Could you check a few things on this drawing? It's one solid part, dimensions in mm from its lowest x, y, z. Coordinates: 2 decimals unless noted, no trailing zeros. Loops run counter-clockwise (first coordinate to the right, second up) from the corner with the lowest first, then second, coordinate; pieces in that order, holes last. Notation, with made-up numbers: M 68,4.5 L 101,4.5 A32 ccw 101,33.5 Z; hole C 60,31 d11. An arc over 180 degrees is marked long. Answer as a JSON object with one key per item and string values. Group by question number.
Item 1: If I drill on line 1 (X direction, y = 26.5, z = 8.5); line 2 (Y direction, x = 201.5, z = 6); line 3 (Z direction, x = 217.5, y = 18.5), over which ranges is the centre line in solid material (lowest first)?
Item 2: Suppose I cut it at A-A (y = 29). Write out the boundary of the cut face in (x, z), then the cut area to 3 significant figures.
Item 3: Suppose I cut it at C-C (x = 96.5). Write out the boundary of the cut face in (y, z), then the cut area to 3 significant figures.
Item 4: Suppose I cut it at B-B (y = 6). Write out the boundary of the cut face in (x, z).
Item 5: Suppose I cut it at D-D (z = 38). Write out the boundary of the cut face in (x, y), then the cut area to 3 significant figures.
Item 6: I'm going to push flat-ended pins straight in: pin 1 Ø3 at (x, y) = (274.5, 12) entering from -Z; pin 2 Ø6 at (x, z) = (151, 66) entering from +Y; pin 3 Ø10 at (x, y) = (83.5, 21.5) entering from +Z. Where does each tip first touch, or does it pass through?
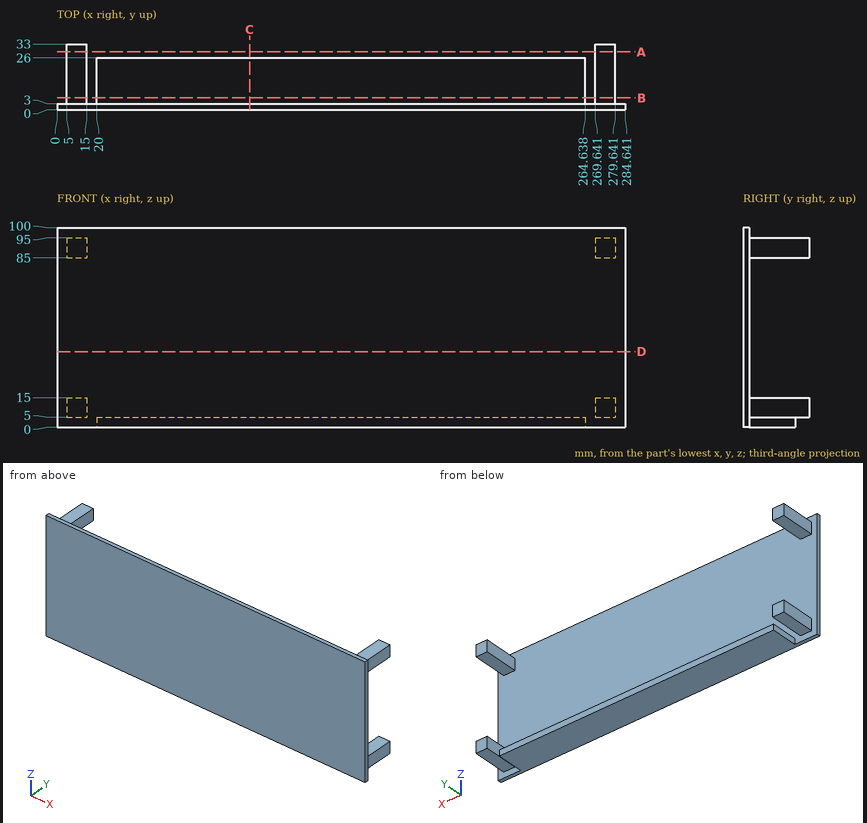
From the geometry:
{
 "1": {"line 1": "5 to 15, 269.64 to 279.64", "line 2": "0 to 3", "line 3": "0 to 5"},
 "2": {"outline": "M 5,5 L 15,5 L 15,15 L 5,15 Z; M 5,85 L 15,85 L 15,95 L 5,95 Z; M 269.64,5 L 279.64,5 L 279.64,15 L 269.64,15 Z; M 269.64,85 L 279.64,85 L 279.64,95 L 269.64,95 Z", "area": "400 mm2"},
 "3": {"outline": "M 0,0 L 26,0 L 26,5 L 3,5 L 3,100 L 0,100 Z", "area": "415 mm2"},
 "4": {"outline": "M 5,5 L 15,5 L 15,15 L 5,15 Z; M 5,85 L 15,85 L 15,95 L 5,95 Z; M 20,0 L 264.64,0 L 264.64,5 L 20,5 Z; M 269.64,5 L 279.64,5 L 279.64,15 L 269.64,15 Z; M 269.64,85 L 279.64,85 L 279.64,95 L 269.64,95 Z"},
 "5": {"outline": "M 0,0 L 284.64,0 L 284.64,3 L 0,3 Z", "area": "854 mm2"},
 "6": {"pin 1": "z = 5", "pin 2": "y = 3", "pin 3": "z = 5"}
}
